Could you check a few things on this model? Use its own coordinates, in mm. Face numbers are marked on the shaded views. A direction names the side the tool comes from. Give positions to 0.01 mm unless a question says otherwise; leave off trailing zeros. Return JSON: item names as keys, results as strings. Group by question number.
1. Please list where these lines run through material, in increasing order: line 1 (X direction, y = -1.2, z = 7); line 2 (Z direction, x = 0.25, y = -2.1); line 3 (Z direction, x = 3.5, y = -4.75).
2. For the marked faces 1 and 2, which set-ups out of +Z, -Z, +X, -X, +Y, -Y let a thin tool reach every point of the face, with its end or its side?
3. If we mould it in two halves opening along X, with no side actions, what happens to the marked faces 3 and 4? For each: +X half, -X half, draft (parallel to the pull), parting line (faces both ways), or undercut.
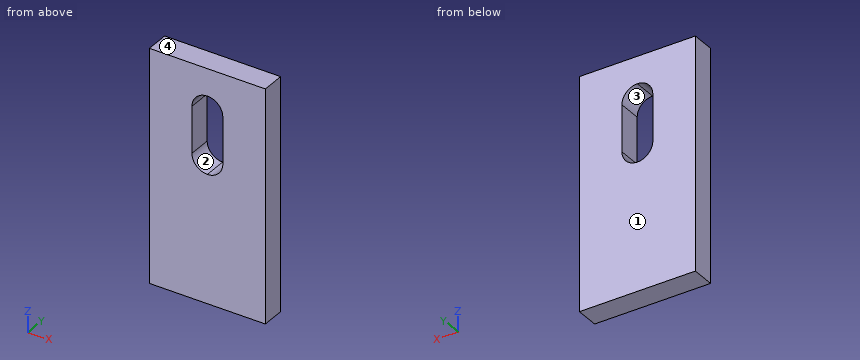
```python
from build123d import *

# Parameters (mm, degrees)
F0_W     = 30
F0_H     = 60
F0_W_2   = 8
F0_H_2   = 20
F1_DEPTH = 6
F2_R     = 3.99999


# Not quite as in the source:
# - a fillet or chamfer is up to 0.001 mm smaller than in the source, because OpenCascade refuses the exact size


with BuildPart() as f1:
    # F0 (on Front) → F1 (new body)
    with BuildSketch(Plane.XZ):
        Rectangle(F0_W, F0_H)
        with Locations((0, 13)):
            Rectangle(F0_W_2, F0_H_2, mode=Mode.SUBTRACT)
    extrude(amount=F1_DEPTH)

    # F2 (radius 4 in the source; OpenCascade refuses exactly that, so slightly less here)
    f2_edges = [f1.edges().sort_by_distance(p)[0] for p in [
        (-4, -3, 23),
        (4, -3, 23),
        (-4, -3, 3),
        (4, -3, 3),
    ]]
    fillet(f2_edges, radius=F2_R)


solid = f1.part
```
Answer:
{
 "1": {"line 1": "x = -15 to -4, 4 to 15", "line 2": "z = -30 to 3.01, 22.99 to 30", "line 3": "z = -30 to 5.06, 20.94 to 30"},
 "2": {"face 1": "+Z, -Z, +X, -X, +Y", "face 2": "+Y, -Y"},
 "3": {"face 3": "undercut", "face 4": "draft"}
}
